from build123d import *

# Parameters (mm, degrees)
F3_DEPTH = 508
F4_R     = 5.08


with BuildPart() as f1:
    # F0 (on Front) → F1 (revolve)
    with BuildSketch(Plane.XZ):
        with BuildLine():
            Line((-32.6849557459, 129.4918209314), (-22.4857572466, 129.4918209314))
            Line((-22.4857572466, 129.4918209314), (-22.4857572466, 8.1203018698))
            ThreePointArc((-22.4857572466, 8.1203018698), (-35.2097717712, -41.1345076384), (6.5492498688, -70.1882667236))
            Line((6.5492498688, -70.1882667236), (6.5492498688, -25.6512276828))
            Line((6.5492498688, -25.6512276828), (6.5492498688, 129.4918209314))
            Line((6.5492498688, 129.4918209314), (6.5492498688, 143.8984274864))
            Line((6.5492498688, 143.8984274864), (-32.6849557459, 143.8984274864))
            Line((-32.6849557459, 143.8984274864), (-51.9365184009, 129.4918209314))
            Line((-51.9365184009, 129.4918209314), (-32.6849557459, 129.4918209314))
        make_face()
    revolve(axis=Axis((6.5492498688, 0, 51.9202966243), (0, 0, -1)))

    # F2 (on face) → F3 (join)
    with BuildSketch(Plane.XY.offset(143.8984274864)):
        Polygon((-12.7665811263, -6.35), (-12.7665811263, 0), (-28.0065811263, 0), align=None)
        Polygon((-12.7665811263, 0), (-12.7665811263, 6.35), (-28.0065811263, 0), align=None)
        Polygon((41.105080864, 0), (25.865080864, 0), (25.865080864, -6.35), align=None)
        Polygon((41.105080864, 0), (25.865080864, 6.35), (25.865080864, 0), align=None)
        Polygon((25.865080864, 0), (25.865080864, 6.35), (-12.7665811263, 6.35), (-12.7665811263, 0), (-12.7665811263, -6.35), (25.865080864, -6.35), align=None)
    extrude(amount=F3_DEPTH)

    # F4
    f4_edges = [f1.edges().sort_by_distance(p)[0] for p in [
        (35.584257, 0, 129.491821),
        (35.584257, 0, 8.120302),
    ]]
    fillet(f4_edges, radius=F4_R)


solid = f1.part
Input: part model. Units: mm. Frame: model coordinates. A direction names the side the tool comes from. Give positions to 0.01 mm unless a question says otherwise; leave off trailing zeros. Write each loop counter-clockwise with the first axis right and the second up, starting at its lowest first coordinate (ties: lowest second). Pieces come first, ordered by that corner, then holes. Notation, with made-up numbers: M 79.25,62 L 127.25,62 A24 ccw 127.25,73 Z; hole C 44.25,29 d6. An arc over 180 degrees is marked long. Use one line per item in the form item = value.
1. Ray query, L1, parallel to Z at x = 41.5, y = 3.5; L2, parallel to Z at x = -22.5, y = -8; L3, parallel to Y at x = 26, z = 470.5. Return the intervals inside material, ascending.
Outcome:
L1 = -53.03 to 1.73, 129.49 to 143.9
L2 = -58.45 to 7.23, 127.56 to 143.9
L3 = -6.29 to 6.29
2. Cut plane A-A on z = 437.5. Return loops of the section in (x, y), and give its area (3 significant figures).
Outcome:
outline = M -28.01,0 L -12.77,-6.35 L 25.87,-6.35 L 41.11,0 L 25.87,6.35 L -12.77,6.35 Z
area = 684 mm²
3. Reachability of faces 4 (the face through (7, 6.35, 394)), 5 (the face through (33.59, 3.13, 394.34)), 6 (the face through (6, -6.35, 394)), 7 (the face through (-20.49, -3.13, 394.34)) from +Z, -Z, +X, -X, +Y, -Y: full face, straight path, thin tool, end or side. Return the list, or none.
Outcome:
face_4 = +Z, +X, -X, +Y
face_5 = +Z, +X, +Y
face_6 = +Z, +X, -X, -Y
face_7 = +Z, -X, -Y
4. First-contact query: P1, Ø12, axis at x = 15, z = 207, coming from the -Y side; P2, Ø8, axis at y = -11, z = 3.5, coming from the +X side; P3, Ø11.5, axis at x = 8, z = 276.5, coming from the +Y side. Flat tips, straight axial feed; report the tip coordinate or a pass-through.
Outcome:
P1 = -6.35
P2 = 41.85
P3 = 6.35
5. Mould query, pull axis Z, two halves, no side actions, for faces 1 (the face through (-20.28, 3.22, 394.34)), 2 (the face through (-19, -25, 129.492)), 3 (the face through (6, -8, 143.898)). Classes: released by +Z, released by -Z, zero draft, split by the parting line, or undercut.
Outcome:
face_1 = zero draft
face_2 = undercut
face_3 = released by +Z
